Could you check a few things on this model? Use its own coordinates, in mm. Coordinates: 2 decimals unless noted, no trailing zeros.
```python
from build123d import *

# Parameters (mm, degrees)
F0_W     = 300
F0_H     = 24.5
F0_R     = 2.65
F1_DEPTH = 2
F2_DEPTH = 10
F3_DEPTH = 30
F4_R     = 1.7
F5_DEPTH = 2
F6_R     = 1.25
F7_DEPTH = 2


with BuildPart() as f1:
    # F0 (on Top) → F1 (new body)
    with BuildSketch(Plane.XY):
        Rectangle(F0_W, F0_H)
        with Locations((-120, 0)):
            Circle(F0_R, mode=Mode.SUBTRACT)
        with Locations((-105, 0)):
            Circle(F0_R, mode=Mode.SUBTRACT)
        with Locations((-90, 0)):
            Circle(F0_R, mode=Mode.SUBTRACT)
        with Locations((-75, 0)):
            Circle(F0_R, mode=Mode.SUBTRACT)
        with Locations((-60, 0)):
            Circle(F0_R, mode=Mode.SUBTRACT)
        with Locations((-45, 0)):
            Circle(F0_R, mode=Mode.SUBTRACT)
        with Locations((-30, 0)):
            Circle(F0_R, mode=Mode.SUBTRACT)
        with Locations((-15, 0)):
            Circle(F0_R, mode=Mode.SUBTRACT)
        Circle(F0_R, mode=Mode.SUBTRACT)
        with Locations((15, 0)):
            Circle(F0_R, mode=Mode.SUBTRACT)
        with Locations((30, 0)):
            Circle(F0_R, mode=Mode.SUBTRACT)
        with Locations((45, 0)):
            Circle(F0_R, mode=Mode.SUBTRACT)
        with Locations((60, 0)):
            Circle(F0_R, mode=Mode.SUBTRACT)
        with Locations((75, 0)):
            Circle(F0_R, mode=Mode.SUBTRACT)
        with Locations((90, 0)):
            Circle(F0_R, mode=Mode.SUBTRACT)
        with Locations((105, 0)):
            Circle(F0_R, mode=Mode.SUBTRACT)
        with Locations((120, 0)):
            Circle(F0_R, mode=Mode.SUBTRACT)
    extrude(amount=F1_DEPTH)

    # F2 (add): a face of the model
    f2_faces = [f1.faces().sort_by_distance(p)[0] for p in [
        (-150, 0, 1),
    ]]
    extrude(f2_faces, amount=F2_DEPTH)

    # F3 (add): a face of the model
    f3_faces = [f1.faces().sort_by_distance(p)[0] for p in [
        (150, 0, 1),
    ]]
    extrude(f3_faces, amount=F3_DEPTH)

    # F4 (on face) → F5 (cut, through all)
    with BuildSketch(Plane.XY.offset(2)):
        with Locations((-153.6, 0)):
            Circle(F4_R)
    extrude(amount=-F5_DEPTH, mode=Mode.SUBTRACT)

    # F6 (on face) → F7 (cut, through all)
    with BuildSketch(Plane.XY.offset(2)):
        with Locations((158.75, -7.25)):
            Circle(F6_R)
    extrude(amount=-F7_DEPTH, mode=Mode.SUBTRACT)


solid = f1.part
```
1. If we mould it in two halves opening along X, with no side actions, what happens to faces 1 (the face through (8, 0, 0)), 2 (the face through (-47.647, 0.117, 0.986))? For each: pulls with the +X half, pulls with the -X half, needs draft (parallel to the pull), parting line crosses it, or undercut.
Verdict:
face 1: needs draft
face 2: undercut
2. I want a section at A-A on z = 0.3. Give the number of separate pieces and of enclosed holes in the cut face, plus the area to 3 significant figures.
Verdict:
separate pieces: 1
enclosed holes: 19
area: 7,940 mm2
3. Please list where these lines run through material, in increasing order: line 1 along Y through (x, z) = (158.75, 0.85); line 2 along Y through (x, z) = (120, 0.85); line 3 along X through (y, z) = (-7.5, 0.15).
Verdict:
line 1: y = -12.25 to -8.5, -6 to 12.25
line 2: y = -12.25 to -2.65, 2.65 to 12.25
line 3: x = -160 to 157.53, 159.97 to 180
